Source: CAD feature listing. Evaluate the final solid. Frame: model axes, mm. A direction names the side the tool comes from. Give positions to 0.01 mm unless a question says otherwise; leave off trailing zeros. Order: outer loops, then holes, each group sorted by start corner. A loop starts at its lowest first (then second) coordinate and runs counter-clockwise, first axis right, second up. Notation, with made-up numbers: M -24,33 L -20,33 A11 ccw -20,39 Z; hole C -27.75,-1.5 d9. An arc over 180 degrees is marked long. Answer as a JSON object with one key per item and string values. Group by question number.
1. Section query D-D (y = 7.25). Output: boundary loops of the cut face in (x, z).
2. Pull-direction query (Z, two-part tool) for faces 3 (the flat face through (-19.33, 1.48, -19.56)), 4 (the cylindrical face through (-5.17, 12.86, 12.47)), 5 (the flat face through (19.33, 1.48, 19.56)); classes: +Z half, -Z half, draft (parallel to the pull), parting line (faces both ways), or undercut.
3. Pin query (flat end, axial travel): P1, Ø3, axis at y = 17.5, z = -16.5, coming from the -X side; P2, Ø4, axis at x = -21.5, z = -2.5, coming from the +Y side; P3, Ø1, axis at x = 7, y = 19.5, coming from the -Z side. Return the tip coordinate at first contact, or that it passes through.
4. Material intervals for L1, parallel to X at y = 12, z = 0; L2, parallel to Y at x = 0, z = 14.7; L3, parallel to Y at x = -2.5, z = 2, sorted ascending. Write a range as [from, to].
5. Section query C-C (y = 15). Output: boundary loops of the cut face in (x, z), plus the area to 3 significant figures.
6. Section query B-B (z = 0). Output: boundary loops of the cut face in (x, y), plus the area to 3 significant figures.
7. Section query A-A (x = 0). Output: boundary loops of the cut face in (y, z).
8. Set-up query: faces 1 (the flat face through (19.56, 1.48, -19.33)), 2 (the flat face through (0, 3, 0)). Return all of +Z, -Z, +X, -X, +Y, -Y with unobstructed straight access to the full face (end or side cutting, diameter ignored); none if empty.
from build123d import *

# Parameters (mm, degrees)
BOSS_EXTRUDE1_DEPTH     = 3
SKETCH4_R               = 16.5
SKETCH4_R_2             = 13.5
BOSS_EXTRUDE2_DEPTH     = 20
CUT_EXTRUDE1_DEPTH      = 46.18296139
CUT_EXTRUDE1_DEPTH_BACK = 46.18296139
SKETCH5_R               = 2.6
CHAMFER1_SIZE           = 5


with BuildPart() as part:
    # Sketch2 → Boss-Extrude1 (new body)
    with BuildSketch(Plane(origin=(0, 0, 0), x_dir=(1, 0, 0), z_dir=(0, 1, 0))):
        Polygon((-11.390872965, 27.5), (-27.5, 11.390872965), (-27.5, -11.390872965), (-11.390872965, -27.5), (11.390872965, -27.5), (27.5, -11.390872965), (27.5, 11.390872965), (11.390872965, 27.5), align=None)
    extrude(amount=BOSS_EXTRUDE1_DEPTH)

    # Sketch4 → Boss-Extrude2 (add)
    with BuildSketch(Plane(origin=(0, 3, 0), x_dir=(1, 0, 0), z_dir=(0, 1, 0))):
        with Locations(Location((0, 0, 0), (0, 0, 270))):
            Circle(SKETCH4_R)
        with Locations(Location((0, 0, 0), (0, 0, 270))):
            Circle(SKETCH4_R_2, mode=Mode.SUBTRACT)
    extrude(amount=BOSS_EXTRUDE2_DEPTH)

    # Sketch5 → Cut-Extrude1 (cut, two sides: drawn at the far end of the back side and taken through both)
    with BuildSketch(Plane.XY.offset(-CUT_EXTRUDE1_DEPTH_BACK)):
        with Locations((0, 15)):
            Circle(SKETCH5_R)
    extrude(amount=CUT_EXTRUDE1_DEPTH + CUT_EXTRUDE1_DEPTH_BACK, mode=Mode.SUBTRACT)

    # Chamfer1
    chamfer1_edges = [part.edges().sort_by_distance(p)[0] for p in [
        (0, 3, -16.5),
    ]]
    chamfer(chamfer1_edges, length=CHAMFER1_SIZE)


solid = part.part
Answer sheet:
{
 "1": {"outline": "C 0,0 d34.5; hole C 0,0 d27"},
 "2": {"face 3": "-Z half", "face 4": "undercut", "face 5": "+Z half"},
 "3": {"P1": "x = -6.87", "P2": "y = 4.86", "P3": "z = -15.17"},
 "4": {"L1": "[-16.5, -13.5], [13.5, 16.5]", "L2": "[0, 12.4], [17.6, 23]", "L3": "[0, 3]"},
 "5": {"outline": "M -2.6,-16.29 L -2.6,-13.25 A13.5 cw -2.6,13.25 L -2.6,16.29 A16.5 ccw Z; M 2.6,-16.29 A16.5 ccw 2.6,16.29 L 2.6,13.25 A13.5 cw 2.6,-13.25 Z", "area": "251 mm^2"},
 "6": {"outline": "M -27.5,0 L 27.5,0 L 27.5,3 L 21.5,3 L 16.5,8 L 16.5,23 L 13.5,23 L 13.5,3 L -13.5,3 L -13.5,23 L -16.5,23 L -16.5,8 L -21.5,3 L -27.5,3 Z", "area": "310 mm^2"},
 "7": {"outline": "M 0,-27.5 L 3,-27.5 L 3,-21.5 L 8,-16.5 L 12.4,-16.5 L 12.4,-13.5 L 3,-13.5 L 3,13.5 L 12.4,13.5 L 12.4,16.5 L 8,16.5 L 3,21.5 L 3,27.5 L 0,27.5 Z; M 17.6,-16.5 L 23,-16.5 L 23,-13.5 L 17.6,-13.5 Z; M 17.6,13.5 L 23,13.5 L 23,16.5 L 17.6,16.5 Z"},
 "8": {"face 1": "-Z, +X, +Y, -Y", "face 2": "+Y"}
}
